Build history of the part. All positions in model axes, mm. A direction names the side the tool comes from. Give positions to 0.01 mm unless a question says otherwise; leave off trailing zeros. Loops run counter-clockwise (first coordinate to the right, second up) from the corner with the lowest first, then second, coordinate; pieces in that order, holes last. Notation, with made-up numbers: M 30.5,-10.75 L 56.5,-10.75 A23 cw 56.5,24.25 Z; hole C 18,-6 d3. An arc over 180 degrees is marked long. Answer as a JSON object with one key per item and string values. Group by question number.
1. Mould opens along X. For faces 1 (the face through (5, -19, -27.185)), 2 (the face through (-11.604, -6.439, 15.916)), 3 (the face through (-16.483, -6.439, 4.791)) say: released by +X, released by -X, zero draft, split by the parting line, or undercut.
2. Drill centre lines: line 1 along Z through (x, y) = (-6, -17); line 2 along Y through (x, z) = (-9.5, -5); line 3 along X through (y, z) = (-2.5, 0). Where is each one in solid material? Low to high. Write a range as [from, to].
3. Drop flat-ended pins along their axis: pin 1 Ø1 at (x, y) = (8, -12) entering from +Z; pin 2 Ø3 at (y, z) = (-33.5, -20.5) entering from -X; pin 3 Ø2 at (x, z) = (0.5, -20.5) entering from +Y. Give the stop position or say it passes through.
4. Slice it at D-D (x = 14). List the corners of the cut face in (y, z), then the cut area to 3 significant figures.
5. Slice it at C-C (z = 9). List the corners of the cut face in (x, y), then the cut area to 3 significant figures.
6. Slice it at B-B (y = -9.5). List the corners of the cut face in (x, z).
7. 3-axis set-ups, long thin cutter, end or side, ignore diameter. For faces 4 (the face through (-11, -12.7, -6)), 5 (the face through (5, -24, -20.835)), 6 (the face through (-22.708, -8, -15)): which of +Z, -Z, +X, -X, +Y, -Y reach the whole face in a straight line?
8. Slice it at A-A (x = -12). List the corners of the cut face in (y, z), then the cut area to 3 significant figures.
from build123d import *

# Parameters (mm, degrees)
F0_W     = 57.15
F0_H     = 44.45
F1_DEPTH = 38.1
F3_DEPTH = 50.8
F4_R     = 5.1343253719
F5_DEPTH = 50.8
F6_R     = 5.1343253719
F7_DEPTH = 25.4
F9_DEPTH = 25.4


with BuildPart() as f1:
    # F0 (on Front) → F1 (new body)
    with BuildSketch(Plane.XZ):
        with Locations((5.8669857811, -4.9598356709)):
            Rectangle(F0_W, F0_H)
    extrude(amount=F1_DEPTH)

    # F2 (on face) → F3 (cut)
    with BuildSketch(Plane.XZ.offset(38.1)):
        with BuildLine():
            Line((-22.7080142189, 17.2651643291), (-22.7080142189, 4.5651643291))
            ThreePointArc((-22.7080142189, 4.5651643291), (-11.3540071095, 15.9191714386), (0, 4.5651643291))
            ThreePointArc((0, 4.5651643291), (2.2272511589, -8.9513703214), (9.0419857811, -20.8348356709))
            Line((9.0419857811, -20.8348356709), (34.4419857811, -20.8348356709))
            Line((34.4419857811, -20.8348356709), (34.4419857811, 17.2651643291))
            Line((34.4419857811, 17.2651643291), (-22.7080142189, 17.2651643291))
        make_face()
    extrude(amount=-F3_DEPTH, mode=Mode.SUBTRACT)

    # F4 (on face) → F5 (cut)
    with BuildSketch(Plane.XZ.offset(38.1)):
        with Locations((-11.3540071095, 4.5651643291)):
            Circle(F4_R)
    extrude(amount=-F5_DEPTH, mode=Mode.SUBTRACT)

    # F6 (on face) → F7 (cut)
    with BuildSketch(Plane.XZ.offset(38.1)):
        with BuildLine():
            Line((-22.7080142189, -20.8348356709), (9.0419857811, -20.8348356709))
            ThreePointArc((9.0419857811, -20.8348356709), (2.2272511589, -8.9513703214), (0, 4.5651643291))
            ThreePointArc((0, 4.5651643291), (-11.3540071095, 15.9191714386), (-22.7080142189, 4.5651643291))
            Line((-22.7080142189, 4.5651643291), (-22.7080142189, -20.8348356709))
        make_face()
        with Locations((-11.3540071095, 4.5651643291)):
            Circle(F6_R, mode=Mode.SUBTRACT)
    extrude(amount=-F7_DEPTH, mode=Mode.SUBTRACT)

    # F8 (on face) → F9 (cut)
    with BuildSketch(Plane.XY.offset(-20.8348356709)):
        with BuildLine():
            ThreePointArc((-15.6066697437, -38.1), (-20.4472184025, -36.0749113012), (-22.7080142189, -31.3398613719))
            Line((-22.7080142189, -31.3398613719), (-22.7080142189, -38.1))
            Line((-22.7080142189, -38.1), (-15.6066697437, -38.1))
        make_face()
        with BuildLine():
            ThreePointArc((34.4419857811, -32.7223523103), (32.5917045845, -36.3084613898), (28.9758909494, -38.1))
            Line((28.9758909494, -38.1), (34.4419857811, -38.1))
            Line((34.4419857811, -38.1), (34.4419857811, -32.7223523103))
        make_face()
    extrude(amount=-F9_DEPTH, mode=Mode.SUBTRACT)


solid = f1.part
Established:
{
 "1": {"face 1": "zero draft", "face 2": "split by the parting line", "face 3": "undercut"},
 "2": {"line 1": "z = [-27.18, -20.83]", "line 2": "y = [-12.7, 0]", "line 3": "x = [-22.71, -13.7], [-9, 0.2]"},
 "3": {"pin 1": "stops at z = -18.88", "pin 2": "stops at x = -22.62", "pin 3": "stops at y = 0"},
 "4": {"outline": "M -38.1,-27.18 L 0,-27.18 L 0,-20.83 L -38.1,-20.83 Z", "area": "242 mm^2"},
 "5": {"outline": "M -21.81,-12.7 L -13.94,-12.7 L -13.94,0 L -21.81,0 Z; M -8.77,-12.7 L -0.9,-12.7 L -0.9,0 L -8.77,0 Z", "area": "200 mm^2"},
 "6": {"outline": "M -22.71,-27.18 L 34.44,-27.18 L 34.44,-20.83 L 9.04,-20.83 A38.54 cw 0,4.57 A11.35 ccw -22.71,4.57 Z; hole C -11.35,4.57 d10.27"},
 "7": {"face 4": "+Z, +X, -X, -Y", "face 5": "+Z, +X, -Y", "face 6": "+Z, -Z, -X, +Y, -Y"},
 "8": {"outline": "M -38.1,-27.18 L 0,-27.18 L 0,-0.53 L -12.7,-0.53 L -12.7,-20.83 L -38.1,-20.83 Z; M -12.7,9.66 L 0,9.66 L 0,15.9 L -12.7,15.9 Z", "area": "579 mm^2"}
}
